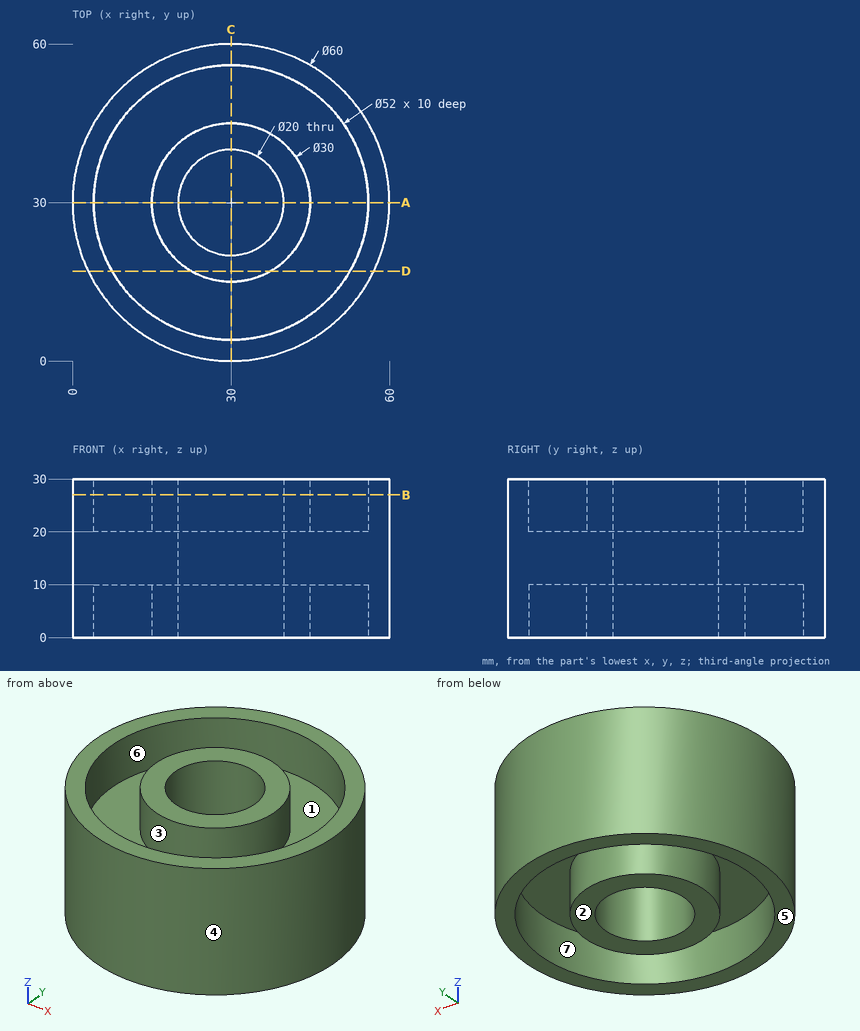
Job drawing, mm, ordinate dimensions from the low corner. One solid piece. A direction names the side the tool comes from. Round coordinates to 2 decimals unless told otherwise and drop trailing zeros. Loops run counter-clockwise (first coordinate to the right, second up) from the corner with the lowest first, then second, coordinate; pieces in that order, holes last.
Item 1: Drill centre lines: line 1 (Y direction, x = 30, z = 8.5); line 2 (X direction, y = 17.5, z = 24.25); line 3 (X direction, y = 38, z = 6.25). Where is each one in solid material? Low to high.
Item 2: Cut at B-B, the plane z = 27. Give the cut face in (x, y), then the cut area to 3 significant figures.
Item 3: Mould opens along X. For the marked faces 1, 2, 3 and 4 say: +X half, -X half, draft (parallel to the pull), parting line (faces both ways), or undercut.
Item 4: 3-axis set-ups, long thin cutter, end or side, ignore diameter. For the marked faces 5, 6 and 7: which of +Z, -Z, +X, -X, +Y, -Y reach the whole face in a straight line?
Item 5: Cut at D-D, the plane y = 17. Give the cut face in (x, z).
Item 6: Drop flat-ended pins along their axis: P1, Ø3, axis at x = 27, z = 7.5, coming from the +Y side; P2, Ø2, axis at x = 44.5, y = 44, coming from the -Z side; P3, Ø10, axis at x = 8, z = 12.5, coming from the -Y side. Give the stop position or say it passes through.
Item 7: Cut at A-A, the plane y = 30. Give the cut face in (x, z).
A:
1. line 1: y = 0 to 4, 15 to 20, 40 to 45, 56 to 60
1. line 2: x = 2.73 to 7.2, 21.71 to 38.29, 52.8 to 57.27
1. line 3: x = 1.09 to 5.26, 17.31 to 24, 36 to 42.69, 54.74 to 58.91
2. outline: circle Ø60 at (30, 30); circle Ø30 at (30, 30); hole circle Ø52 at (30, 30); hole circle Ø20 at (30, 30)
2. area: 1,100 mm2
3. face 1: undercut
3. face 2: draft
3. face 3: undercut
3. face 4: parting line
4. face 5: -Z, +X, -X, +Y, -Y
4. face 6: +Z
4. face 7: -Z
5. outline: (2.96, 0) - (7.48, 0) - (7.48, 10) - (22.52, 10) - (22.52, 0) - (37.48, 0) - (37.48, 10) - (52.52, 10) - (52.52, 0) - (57.04, 0) - (57.04, 30) - (52.52, 30) - (52.52, 20) - (37.48, 20) - (37.48, 30) - (22.52, 30) - (22.52, 20) - (7.48, 20) - (7.48, 30) - (2.96, 30) - close
6. P1: stops at y = 59.96
6. P2: stops at z = 10
6. P3: stops at y = 5.28
7. outline: (0, 0) - (4, 0) - (4, 10) - (15, 10) - (15, 0) - (20, 0) - (20, 30) - (15, 30) - (15, 20) - (4, 20) - (4, 30) - (0, 30) - close; (40, 0) - (45, 0) - (45, 10) - (56, 10) - (56, 0) - (60, 0) - (60, 30) - (56, 30) - (56, 20) - (45, 20) - (45, 30) - (40, 30) - close
